Could you check a few things on this model? Use its own coordinates, in mm. A direction names the side the tool comes from. Give positions to 0.01 mm unless a question says otherwise; leave off trailing zeros. Write each loop counter-clockwise with the first axis right and the second up, starting at its lowest first coordinate (ties: lowest second). Pieces come first, ordered by that corner, then holes. Notation, with made-up numbers: M -17.5,39 L -5.5,39 A22 ccw -5.5,56 Z; hole C 89.25,72 d10. An arc over 180 degrees is marked long. One line per item, written item: value.
```python
from build123d import *

# Parameters (mm, degrees)
SKETCH1_R            = 47.625
BOSS_EXTRUDE1_DEPTH  = 3.81
BOSS_EXTRUDE2_START  = 12.7
SKETCH4_R            = 47.625
SKETCH4_R_2          = 44.45
BOSS_EXTRUDE2_DEPTH  = 12.7
SKETCH7_W            = 88.9
SKETCH7_H            = 1.778
BOSS_EXTRUDE14_DEPTH = 5.08


with BuildPart() as part:
    # Sketch1 → Boss-Extrude1 (new body)
    with BuildSketch(Plane.XY):
        with Locations(Location((0, 0, 0), (0, 0, 180))):
            Circle(SKETCH1_R)
    extrude(amount=BOSS_EXTRUDE1_DEPTH)

    # Sketch4 → Boss-Extrude2 (add)
    with BuildSketch(Plane(origin=(0, 0, 0), x_dir=(-1, 0, 0), z_dir=(0, 0, -1)).offset(BOSS_EXTRUDE2_START)):
        Circle(SKETCH4_R)
        with Locations(Location((0, 0, 0), (0, 0, 180))):
            Circle(SKETCH4_R_2, mode=Mode.SUBTRACT)
    extrude(amount=-BOSS_EXTRUDE2_DEPTH)

    # Sketch7 → Boss-Extrude14 (add)
    with BuildSketch(Plane(origin=(0, 0, 0), x_dir=(-1, 0, 0), z_dir=(0, 0, -1))):
        with Locations((-0.004601407, -1.528565374)):
            Rectangle(SKETCH7_W, SKETCH7_H)
    extrude(amount=BOSS_EXTRUDE14_DEPTH)


solid = part.part
```
1) If we section it at D-D, the plane z = -8.25: Write out the boundary of the cut face in (x, y) (3 decimals), then the cut area to 3 significant figures.
Outcome:
outline: C 0,0 d95.25; hole C 0,0 d88.9
area: 918 mm^2
2) If we section it at B-B, the plane x = 0: Write out the boundary of the cut face in (y, z) (3 decimals).
Outcome:
outline: M -47.625,-12.7 L -44.45,-12.7 L -44.45,0 L -2.418,0 L -2.418,-5.08 L -0.64,-5.08 L -0.64,0 L 44.45,0 L 44.45,-12.7 L 47.625,-12.7 L 47.625,3.81 L -47.625,3.81 Z
3) On a 3-axis mill with a long thin cutter (end or side, diameter ignored), from which of +Z, -Z, +X, -X, +Y, -Y can I reach the whole of each face in a straight line? I mean faces 1 (the face through (1, -1, 3.81)), 2 (the face through (1, -19, 0)). Say none if no direction works.
Outcome:
face 1: +Z, +X, -X, +Y, -Y
face 2: -Z
4) I'm going to push flat-ended pins straight in: pin 1 (2.5 mm diameter, centred on x = -21.5, z = -2, fed in from +Y); pin 2 (5 mm diameter, centred on x = 33.5, z = -9.5, fed in from -Y); pin 3 (4 mm diameter, centred on x = 22, z = -1.5, fed in from -Y). Where does each tip first touch, or does it pass through?
Outcome:
pin 1: stops at y = 43.11
pin 2: stops at y = -36.15
pin 3: stops at y = -43.22
5) Please list where these lines run through material, in increasing order: L1, parallel to Y at x = 0, z = -3.5 (3 decimals); L2, parallel to Y at x = -12.5, z = -2.5; L3, parallel to Y at x = 0, z = -9 (3 decimals). Write a range as from..to.
Outcome:
L1: y = -47.625..-44.45, -2.418..-0.64, 44.45..47.625
L2: y = -45.96..-42.66, -2.42..-0.64, 42.66..45.96
L3: y = -47.625..-44.45, 44.45..47.625
6) If we section it at A-A, the plane z = -2.75: Write out the boundary of the cut face in (x, y) (3 decimals), then the cut area to 3 significant figures.
Outcome:
outline: C 0,0 d95.25; hole M -44.445,-0.64 L 44.445,-0.64 A44.45 ccw long Z; hole M -44.384,-2.418 A44.45 ccw 44.384,-2.418 Z
area: 1,080 mm^2
7) We'd pull the mould along Y, two halves only. Please class faces 3 (the face through (-32, -32, -12.7)), 4 (the face through (1, -2.418, -3)), 5 (the face through (42.397, -13.352, -6.439)), 6 (the face through (37.794, -28.979, -4.561)): pulls with the +Y half, pulls with the -Y half, needs draft (parallel to the pull), parting line crosses it, or undercut.
Outcome:
face 3: needs draft
face 4: undercut
face 5: undercut
face 6: parting line crosses it
8) If we section it at C-C, the plane y = -22: Write out the boundary of the cut face in (x, z), then the cut area to 3 significant figures.
Outcome:
outline: M -42.24,-12.7 L -38.62,-12.7 L -38.62,0 L 38.62,0 L 38.62,-12.7 L 42.24,-12.7 L 42.24,3.81 L -42.24,3.81 Z
area: 414 mm^2
